Could you check a few things on this model? Use its own coordinates, in mm. Give positions to 0.01 mm unless a question says otherwise; leave off trailing zeros. Loops run counter-clockwise (first coordinate to the right, second up) from the corner with the lowest first, then second, coordinate; pieces in that order, holes last. Notation, with made-up numbers: M 64,-39 L 111,-39 A23 ccw 111,-26 Z; hole C 80,50 d8. An arc over 180 degrees is marked long. Return JSON: item names as keys, results as strings. Group by question number.
1. Please list where these lines run through material, in increasing order: line 1 (Y direction, x = -707, z = 33); line 2 (X direction, y = -734, z = 3.5); line 3 (X direction, y = -466, z = 28.5).
2. If we section it at C-C (z = 39): Write out the boundary of the cut face in (x, y), plus the area to 3 significant figures.
3. For pin 1 (12 mm diameter, centred on x = -401, z = 17, fed in from -Y); pin 2 (10 mm diameter, centred on x = 261.5, z = 9, fed in from -Y); pin 3 (12 mm diameter, centred on x = -512, z = 41, fed in from +Y), each with a flat end and sliding along its axis, tell me the tip position at first contact or that it passes through.
```python
from build123d import *

# Parameters (mm, degrees)
EXTRUDE_1_DEPTH = 60
CHAMFER3_SIZE2  = 11.912970931
CHAMFER3_SIZE   = 60
CHAMFER4_SIZE2  = 11.912970931
CHAMFER4_SIZE   = 60
CHAMFER5_SIZE2  = 9.519169095
CHAMFER5_SIZE   = 60


with BuildPart() as part:
    # Эскиз1 → Бобышка-Вытянуть1 (new body)
    with BuildSketch(Plane.XY):
        Polygon((-849.589927609, 515.838957491), (787.506047005, 606.405063543), (281.615569427, -953.197537878), align=None)
    extrude(amount=EXTRUDE_1_DEPTH)

    # Chamfer3
    chamfer3_edges = [part.edges().sort_by_distance(p)[0] for p in [
        (-31.041940302, 561.122010517, 60),
    ]]
    chamfer3_side = [part.faces().sort_by_distance(p)[0] for p in [
        (-31.041940302, 561.122010517, 59.761740581),
    ]]
    chamfer(chamfer3_edges, length=CHAMFER3_SIZE - 0.0001, length2=CHAMFER3_SIZE2 - 0.0001, reference=chamfer3_side[0])  # a hair under: the kernel refuses the full size

    # Chamfer4
    chamfer4_edges = [part.edges().sort_by_distance(p)[0] for p in [
        (532.590398399, -179.470785737, 60),
    ]]
    chamfer4_side = [part.faces().sort_by_distance(p)[0] for p in [
        (532.590398399, -179.470785737, 59.761740581),
    ]]
    chamfer(chamfer4_edges, length=CHAMFER4_SIZE - 0.0001, length2=CHAMFER4_SIZE2 - 0.0001, reference=chamfer4_side[0])  # a hair under: the kernel refuses the full size

    # Chamfer5
    chamfer5_edges = [part.edges().sort_by_distance(p)[0] for p in [
        (-283.987179091, -218.679290193, 60),
    ]]
    chamfer5_side = [part.faces().sort_by_distance(p)[0] for p in [
        (-283.987179091, -218.679290193, 59.809616618),
    ]]
    chamfer(chamfer5_edges, length=CHAMFER5_SIZE - 0.0001, length2=CHAMFER5_SIZE2 - 0.0001, reference=chamfer5_side[0])  # a hair under: the kernel refuses the full size


solid = part.part
```
Answer:
{
 "1": {"line 1": "y = 339.25 to 517.17", "line 2": "x = 113.53 to 351.99", "line 3": "x = -87.84 to 433.7"},
 "2": {"outline": "M -836.37,508.81 L 278.2,-938.62 L 776.66,598.05 Z", "area": "1,220,000 mm²"},
 "3": {"pin 1": "stops at y = -70.25", "pin 2": "stops at y = -931.36", "pin 3": "stops at y = 527.6"}
}
